Work out the finished part from the listing and answer in its coordinate system (mm). Face numbers are marked on the shaded views. A direction names the side the tool comes from. Coordinates: 2 decimals unless noted, no trailing zeros. Order: outer loops, then holes, each group sorted by start corner. A loop starts at its lowest first (then second) coordinate and runs counter-clockwise, first axis right, second up. Notation, with made-up numbers: M 32.5,-22 L 89.5,-22 A22 cw 89.5,-1 Z; hole C -34,5 d7. An arc over 180 degrees is marked long. Answer in a Markdown table with one row per item. Add a question column.
Item 1: The part is cut by section C-C (z = -2.5). Write down the section's boundary in (x, y) (3 decimals), then the cut area to 3 significant figures.
Item 2: The part is cut by section A-A (x = 6.75). Write down the section's boundary in (y, z) (1 decimal), then the cut area to 3 significant figures.
Item 3: Consider line 1 (Y direction, x = 2.5, z = -12.75) (3 decimals); line 2 (Z direction, x = 1.25, y = 10.5) (3 decimals); line 3 (Z direction, x = 8.75, y = 7) (1 decimal). Determine where each line is inside the solid, lowest interval first. Write a range as from..to.
Item 4: The part is cut by section B-B (y = 2). Write down the section's boundary in (x, z).
Item 5: Flat-ended cylindrical pins translate along their axes: pin 1 Ø0.8 at (y, z) = (7.5, -20) entering from +X; pin 2 Ø1.9 at (x, y) = (2, 5.5) entering from -Z; pin 3 Ø1.9 at (x, y) = (5, 8) entering from +Z (3 decimals); pin 4 Ø5 at (x, y) = (6, 8) entering from -Z. Find the tip coordinate at first contact, or state that the pin passes through.
Item 6: Which of the six approach directions +Z, -Z, +X, -X, +Y, -Y give full straight-line access (tool end or side, diameter ignored) to the marked faces 1, 2, 3, 4 and 5?
Item 7: The mould has two halves that part along X. Classify the marked faces 6, 7 and 8: released by +X, released by -X, zero draft, split by the parting line, or undercut.
Item 8: The part is cut by section D-D (x = 2.5). Write down the section's boundary in (y, z) (3 decimals).
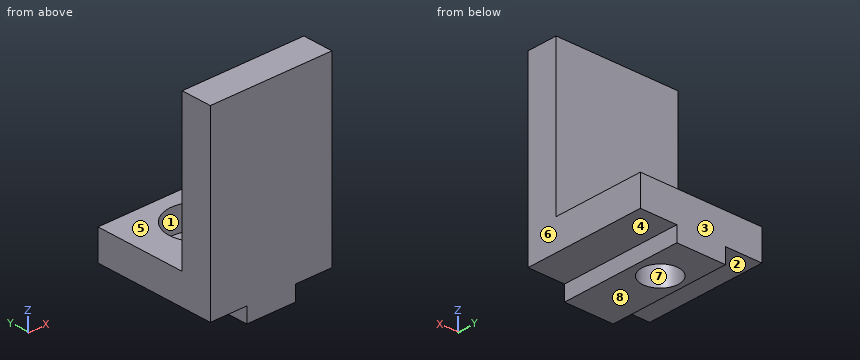
Autodesk Inventor part; units mm, degrees
ref_plane "YZ Plane" through (0, 0, 0) normal (1, 0, 0) x (0, 1, 0)
ref_plane "XZ Plane" through (0, 0, 0) normal (0, 1, 0) x (-1, 0, 0)
ref_plane "XY Plane" through (0, 0, 0) normal (0, 0, 1) x (1, 0, 0)
sketch "Sketch1" plane through (0, 0, 0) normal (1, 0, 0) x (0, 1, 0)
  line L0 (0, 0) -> (0, -19.05)
  line L1 (0, -19.05) -> (12.7, -19.05)
  line L2 (12.7, -19.05) -> (12.7, -15.875)
  line L3 (12.7, -15.875) -> (3.175, -15.875)
  line L4 (3.175, -15.875) -> (3.175, 0)
  line L5 (3.175, 0) -> (0, 0)
  dimension "d0" = 3.175
  dimension "d1" = 12.7
  dimension "d4" = 3.175
  dimension "d5" = 19.05
extrude "Extrusion1" add sketch "Sketch1" along normal blind 12.7
sketch "Sketch4" plane through (0, 0, -19.05) normal (0, 0, -1) x (-1, 0, 0)
  line L0 (0, 12.7) -> (-12.7, 12.7)
  line L1 (0, 0) -> (-12.7, 0)
  line L2 (-8.89, 12.7) -> (-3.81, 12.7)
  line L3 (-3.81, 12.7) -> (-3.81, 0)
  line L4 (-3.81, 0) -> (-8.89, 0)
  line L5 (-8.89, 0) -> (-8.89, 12.7)
  line L6 (0, 0) -> (0, 12.7)
  line L7 (0, 12.7) -> (-12.7, 12.7)
  line L8 (-12.7, 0) -> (-12.7, 12.7)
  line L9 (0, 0) -> (-12.7, 0)
  dimension "d22" = 5.08
  dimension "d23" = 12.7
  dimension "d24" = 3.81
extrude "Extrusion2" add sketch "Sketch4" along normal blind 1.5875 contours L3 L1 L5 L0
sketch "Sketch5" plane through (0, 3.175, -15.875) normal (0, 0, 1) x (1, 0, 0)
  line L0 (0, 9.525) -> (0, 0)
  line L1 (0, 0) -> (12.7, 0)
  line L2 (12.7, 9.525) -> (12.7, 0)
  line L3 (0, 9.525) -> (12.7, 9.525)
  point P0 (0, -3.175)
  point P1 (6.2739, 4.8175)
hole "Hole3" at (6.2739, 7.9925, -15.875) direction (0, 0, -1) diameter 3.81 end through all counterbore diameter 6.35 counterbore depth 2.54
equation "\"d4\" = d0"
equation "\"d24\" = -0.5 * d22 + 0.5 * d23"
properties part number "spring tab for on arm"
Reply:
| question | item | result |
|---|---|---|
| 1 | outline | M 0,0 L 12.7,0 L 12.7,3.175 L 0,3.175 Z |
| 1 | area | 40.3 mm2 |
| 2 | outline | M 0,-20.6 L 6.1,-20.6 L 6.1,-18.4 L 4.9,-18.4 L 4.9,-15.9 L 3.2,-15.9 L 3.2,0 L 0,0 Z; M 9.8,-20.6 L 12.7,-20.6 L 12.7,-15.9 L 11.1,-15.9 L 11.1,-18.4 L 9.8,-18.4 Z |
| 2 | area | 86.7 mm2 |
| 3 | line 1 | y = 0..3.175 |
| 3 | line 2 | z = -19.05..-15.875 |
| 3 | line 3 | z = -20.6..-18.4 |
| 4 | outline | M 0,-19.05 L 3.81,-19.05 L 3.81,-20.64 L 8.89,-20.64 L 8.89,-19.05 L 12.7,-19.05 L 12.7,0 L 0,0 Z |
| 5 | pin 1 | stops at x = 8.89 |
| 5 | pin 2 | stops at z = -19.05 |
| 5 | pin 3 | stops at z = -18.415 |
| 5 | pin 4 | stops at z = -20.64 |
| 6 | face 1 | +Z |
| 6 | face 2 | -Z, -X, +Y, -Y |
| 6 | face 3 | +Z, -Z, +X, -X, +Y |
| 6 | face 4 | -Z, +X, +Y, -Y |
| 6 | face 5 | +Z, +X, -X, +Y |
| 7 | face 6 | released by +X |
| 7 | face 7 | undercut |
| 7 | face 8 | zero draft |
| 8 | outline | M 0,-19.05 L 12.7,-19.05 L 12.7,-15.875 L 3.175,-15.875 L 3.175,0 L 0,0 Z |
